Part model, mm, in its own coordinate system. Face numbers are marked on the shaded views. Give positions to 0.01 mm unless a question says otherwise; leave off trailing zeros. Loops run counter-clockwise (first coordinate to the right, second up) from the corner with the lowest first, then second, coordinate; pieces in that order, holes last. Notation, with made-up numbers: M 4,-31.5 L 42,-31.5 A12 cw 42,-12.5 Z; hole C -35,21 d4. An arc over 180 degrees is marked long. Answer in a Markdown table with one row per item.
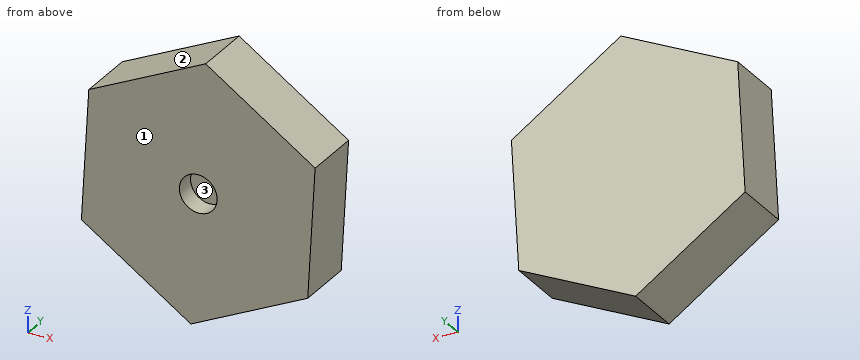
from build123d import *

# Parameters (mm, degrees)
BOSS_EXTRUDE1_DEPTH = 38.1
SKETCH2_R           = 12.7
CUT_EXTRUDE1_DEPTH  = 12.7


with BuildPart() as part:
    # Sketch1 → Boss-Extrude1 (new body)
    with BuildSketch(Plane(origin=(0, 0, 0), x_dir=(1, 0, 0), z_dir=(0, 1, 0))):
        Polygon((73.594904868, 48.225615366), (-4.967155586, 87.847864888), (-78.562060454, 39.622249522), (-73.594904868, -48.225615366), (4.967155586, -87.847864888), (78.562060454, -39.622249522), align=None)
    extrude(amount=BOSS_EXTRUDE1_DEPTH)

    # Sketch2 → Cut-Extrude1 (cut)
    with BuildSketch(Plane.XZ):
        Circle(SKETCH2_R)
    extrude(amount=-CUT_EXTRUDE1_DEPTH, mode=Mode.SUBTRACT)


solid = part.part
(1) Pull direction Z, two halves, no side cores. Call the marked faces 1, 2 and 3: +Z half, -Z half, draft (parallel to the pull), parting line (faces both ways), or undercut.
Recorded:
| item | result |
|---|---|
| face 1 | draft |
| face 2 | +Z half |
| face 3 | undercut |
(2) Pin check, flat tips, straight feed: pin 1 Ø6 at (x, y) = (-45, 18) entering from -Z; pin 2 Ø2 at (x, z) = (46.5, -22) entering from -Y; pin 3 Ø3 at (y, z) = (29.5, -48.5) entering from +X; pin 4 Ø6 at (x, y) = (22, 12) entering from +Z. Stop position of each tip, or through.
Recorded:
| item | result |
|---|---|
| pin 1 | stops at z = -63.58 |
| pin 2 | stops at y = 0 |
| pin 3 | stops at x = 73.66 |
| pin 4 | stops at z = 78.65 |
(3) Saw through at C-C (z = 0). Write the cut outline in (x, y).
Recorded:
| item | result |
|---|---|
| outline | M -76.32,0 L -12.7,0 L -12.7,12.7 L 12.7,12.7 L 12.7,0 L 76.32,0 L 76.32,38.1 L -76.32,38.1 Z |
(4) Drill centre lines: line 1 along Z through (x, y) = (0, 9); line 2 along X through (y, z) = (7, 80); line 3 along X through (y, z) = (12.5, -25). Where is each one in solid material? Low to high.
Recorded:
| item | result |
|---|---|
| line 1 | z = -85.34 to -12.7, 12.7 to 85.34 |
| line 2 | x = -10.59 to 16.94 |
| line 3 | x = -77.74 to 74.91 |
(5) Saw through at D-D (x = 0). Write the cut outline in (y, z).
Recorded:
| item | result |
|---|---|
| outline | M 0,-85.34 L 38.1,-85.34 L 38.1,85.34 L 0,85.34 L 0,12.7 L 12.7,12.7 L 12.7,-12.7 L 0,-12.7 Z |
(6) Saw through at B-B (y = 31). Write the cut outline in (x, z).
Recorded:
| item | result |
|---|---|
| outline | M -78.56,-39.62 L -4.97,-87.85 L 73.59,-48.23 L 78.56,39.62 L 4.97,87.85 L -73.59,48.23 Z |
(7) Saw through at A-A (y = 6.5). Write the cut outline in (x, z).
Recorded:
| item | result |
|---|---|
| outline | M -78.56,-39.62 L -4.97,-87.85 L 73.59,-48.23 L 78.56,39.62 L 4.97,87.85 L -73.59,48.23 Z; hole C 0,0 d25.4 |
